Study the drawing (mm; zero at the part's minimum x, y, z) and answer. A direction names the side the tool comes from. Round coordinates to 2 decimals unless told otherwise and drop trailing zeros. Write each loop counter-clockwise with the first axis right and the second up, starting at its lowest first coordinate (ties: lowest second). Pieces come first, ordered by that corner, then holes. Notation, with made-up numbers: (85.5, 37) - (99.5, 37) arc R7 cw to (99.5, 42) - close; hole circle Ø9 at (-4, 18). An arc over 180 degrees is marked (long way). Return JSON: item names as keys, results as strings. Group by question number.
(1) Which of the six approach directions +Z, -Z, +X, -X, +Y, -Y give full straight-line access (tool end or side, diameter ignored) to the marked faces 5 and 6?
(2) Section D-D, the plane z = 6.25 is taken. Write down the section's boundary in (x, y) (1 decimal), then the cut area to 3 significant figures.
(3) Section B-B, the plane y = 6.5 is taken. Write down the section's boundary in (x, z).
(4) Section A-A, the plane x = 9.5 is taken. Write down the section's boundary in (y, z), then the cut area to 3 significant figures.
(5) Determine the mould class of the marked faces 1, 2, 3 and 4 for opening direction Z: +Z half, -Z half, draft (parallel to the pull), parting line (faces both ways), or undercut.
(6) Each of these flat-tipped pins is pushed along its axis until it touches: pin 1 (6 mm diameter, centred on y = 13, z = 11.5, fed in from -X); pin 2 (6 mm diameter, centred on y = 6, z = 20.5, fed in from -X); pin 3 (1.5 mm diameter, centred on x = 4, y = 6, fed in from +Z). Where does it stop, or does it pass through?
(7) Find the intervals of material crossed by line 1 along X through (y, z) = (4.75, 4.75); line 2 along Z through (x, y) = (4.25, 10) (1 decimal); line 3 along Y through (x, z) = (13.5, 16.75), in increasing order. Write a range as [from, to].
(8) Section C-C, the plane x = 4.25 is taken. Write down the section's boundary in (y, z).
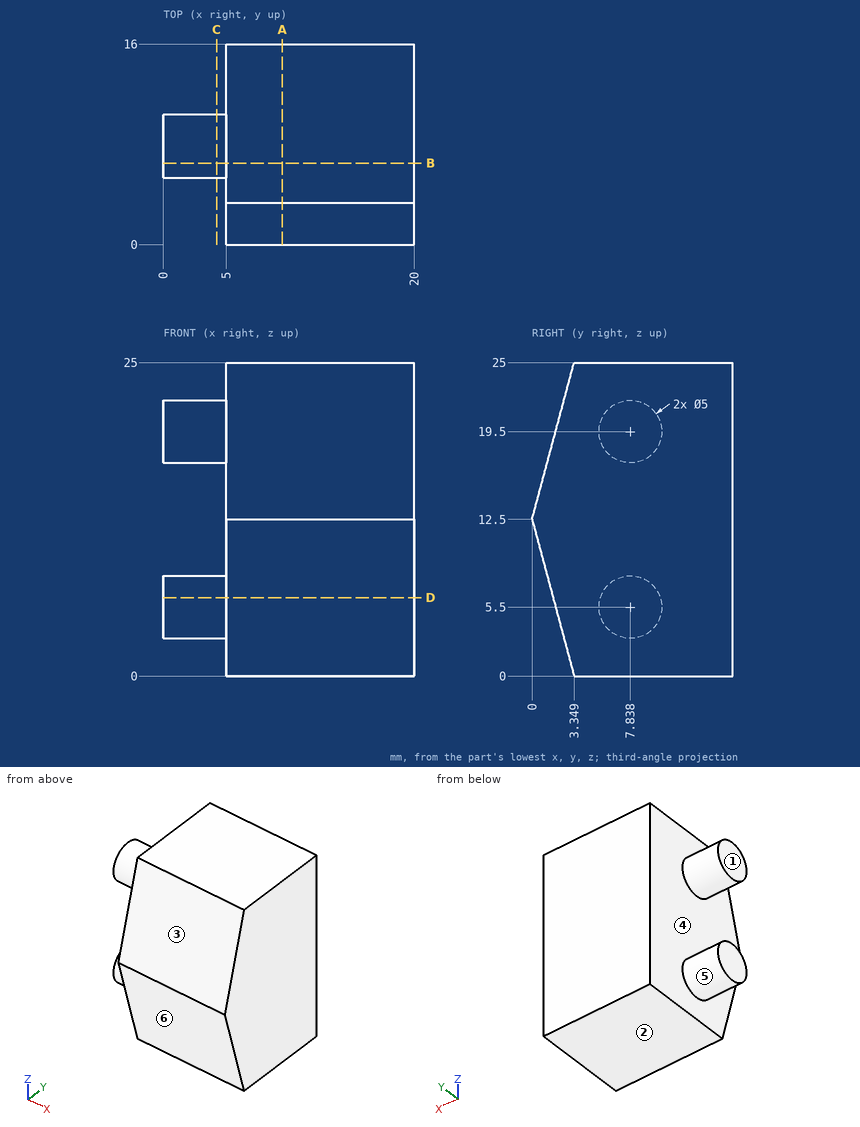
Working result:
{
 "1": {"face 5": "-X", "face 6": "-Z, +X, -X, -Y"},
 "2": {"outline": "(0, 5.5) - (5, 5.5) - (5, 1.7) - (20, 1.7) - (20, 16) - (5, 16) - (5, 10.2) - (0, 10.2) - close", "area": "239 mm^2"},
 "3": {"outline": "(0, 3.39) - (5, 3.39) - (5, 0) - (20, 0) - (20, 25) - (5, 25) - (5, 21.61) - (0, 21.61) - (0, 17.39) - (5, 17.39) - (5, 7.61) - (0, 7.61) - close"},
 "4": {"outline": "(0, 12.5) - (3.35, 0) - (16, 0) - (16, 25) - (3.35, 25) - close", "area": "358 mm^2"},
 "5": {"face 1": "draft", "face 2": "-Z half", "face 3": "+Z half", "face 4": "undercut"},
 "6": {"pin 1": "stops at x = 5", "pin 2": "stops at x = 0", "pin 3": "stops at z = 21.75"},
 "7": {"line 1": "x = [5, 20]", "line 2": "z = [4.2, 6.8], [18.2, 20.8]", "line 3": "y = [1.14, 16]"},
 "8": {"outline": "circle Ø5 at (7.84, 5.5); circle Ø5 at (7.84, 19.5)"}
}
